from build123d import *

# Parameters (mm, degrees)
F0_W     = 76
F0_H     = 36
F1_DEPTH = 700


# Not quite as in the source:
# - ends of sketch curves that miss each other by under 0.0002 mm in the source are joined


with BuildPart() as f1:
    # F0 (on Front) → F1 (new body)
    with BuildSketch(Plane.XZ):
        with BuildLine():
            ThreePointArc((-37.999999, 20), (-39.4142135624, 19.4142135624), (-40, 17.999999))
            Line((-40, 17.999999), (-40, -18))
            ThreePointArc((-40, -18), (-39.4142128553, -19.4142142695), (-37.999999, -20))
            Line((-37.999999, -20), (38, -20))
            ThreePointArc((38, -20), (39.4142139159, -19.4142132088), (40, -18))
            Line((40, -18), (40, 18))
            ThreePointArc((40, 18), (39.4142139159, 19.4142132088), (38.000001, 20))
            Line((38.000001, 20), (-37.999999, 20))
        make_face()
        Rectangle(F0_W, F0_H, mode=Mode.SUBTRACT)
    extrude(amount=F1_DEPTH)


solid = f1.part
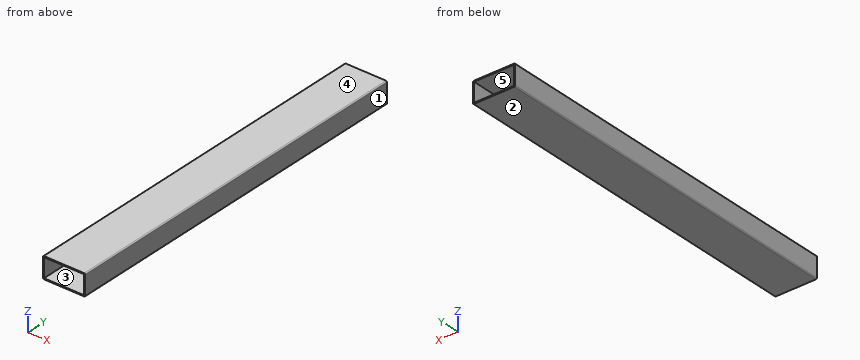
Here's how the part is built. I have some questions about the finished solid (model axes, mm). Face numbers are marked on the shaded views. A direction names the side the tool comes from. Round coordinates to 2 decimals unless told otherwise and drop trailing zeros. Loops run counter-clockwise (first coordinate to the right, second up) from the corner with the lowest first, then second, coordinate; pieces in that order, holes last.
1. If we section it at A-A on x = -18.5: Write out the boundary of the cut face in (y, z).
Answer list:
outline: (-700, -20) - (0, -20) - (0, -18) - (-700, -18) - close; (-700, 18) - (0, 18) - (0, 20) - (-700, 20) - close
2. If we section it at C-C on z = 10: Write out the boundary of the cut face in (x, y), plus the area to 3 significant figures.
Answer list:
outline: (-40, -700) - (-38, -700) - (-38, 0) - (-40, 0) - close; (38, -700) - (40, -700) - (40, 0) - (38, 0) - close
area: 2,800 mm2
3. If we section it at B-B on y = -296: Write out the boundary of the cut face in (x, z).
Answer list:
outline: (-40, -18) arc R2 ccw to (-38, -20) - (38, -20) arc R2 ccw to (40, -18) - (40, 18) arc R2 ccw to (38, 20) - (-38, 20) arc R2 ccw to (-40, 18) - close; hole (-38, -18) - (38, -18) - (38, 18) - (-38, 18) - close
4. We'd pull the mould along Z, two halves only. Please class the marked faces 1, 2 and 3: +Z half, -Z half, draft (parallel to the pull), parting line (faces both ways), or undercut.
Answer list:
face 1: draft
face 2: -Z half
face 3: undercut
5. Which directions (+Z, -Z, +X, -X, +Y, -Y) give clear straight access to the entire face, cutting with the end or side of a thin tool? Please do the marked faces 4 and 5.
Answer list:
face 4: +Z, +X, -X, +Y, -Y
face 5: +Y, -Y
6. If I drill on line 1 along Z through (x, y) = (-4, -549.5); line 2 along X through (y, z) = (-390, 15), over which ranges is the centre line in solid material (lowest first)?
Answer list:
line 1: z = -20 to -18, 18 to 20
line 2: x = -40 to -38, 38 to 40
